Check sheet for the modelled part. Datum: model origin and axes. Units: mm. Face numbers are marked on the shaded views. Coordinates: 2 decimals unless noted, no trailing zeros. Loops run counter-clockwise (first coordinate to the right, second up) from the corner with the lowest first, then second, coordinate; pieces in that order, holes last.
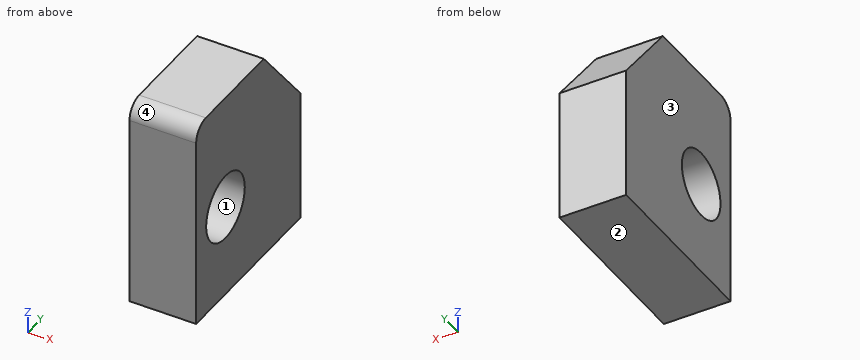
from build123d import *

# Parameters (mm, degrees)
F0_R     = 12.7
F1_DEPTH = 25.4


with BuildPart() as f1:
    # F0 (on Right) → F1 (new body)
    with BuildSketch(Plane.YZ):
        with BuildLine():
            Line((-8.451596, 44.603311), (-46.551596, 44.603311))
            ThreePointArc((-46.551596, 44.603311), (-51.041724, 42.743439), (-52.901596, 38.253311))
            Line((-52.901596, 38.253311), (-52.901596, -35.611195))
            Line((-52.901596, -35.611195), (15.764037, -35.611195))
            Line((15.764037, -35.611195), (15.764037, 15.188805))
            Line((15.764037, 15.188805), (-8.451596, 44.603311))
        make_face()
        with Locations((-33.608079, 0)):
            Circle(F0_R, mode=Mode.SUBTRACT)
    extrude(amount=F1_DEPTH)


solid = f1.part
(1) Gauge pin test, flat ends, axial feed: P1, Ø4, axis at y = 4.5, z = 21, coming from the -X side; P2, Ø20.5, axis at y = -33.61, z = 0, coming from the +X side. Record the tip position at first contact, or that the pin passes through.
(2) Section check D-D, the plane z = 35.5. Enter the section's corners in (x, y), plus the area to 3 significant figures.
(3) Section check B-B, the plane x = 1.75. Enter the section's corners in (y, z), plus the area to 3 significant figures.
(4) Section check A-A, the plane z = 0. Enter the section's corners in (x, y), plus the area to 3 significant figures.
(5) Section check C-C, the plane y = -35.5. Enter the section's corners in (x, z), plus the area to 3 significant figures.
(6) Draft check along Z on the marked faces 1, 2, 3 and 4. Enter one of: pulls with the +Z half, pulls with the -Z half, needs draft (parallel to the pull), parting line crosses it, or undercut.
(7) Scan lines: line 1 along Z through (x, y) = (18.25, -33); line 2 along Z through (x, y) = (12.25, -43); line 3 along Y through (x, z) = (12.5, -2). Record each from-to range of solid material in increasing order.
Determined:
1. P1: stops at x = 0
1. P2: passes through
2. outline: (0, -52.9) - (25.4, -52.9) - (25.4, -0.96) - (0, -0.96) - close
2. area: 1,320 mm2
3. outline: (-52.9, -35.61) - (15.76, -35.61) - (15.76, 15.19) - (-8.45, 44.6) - (-46.55, 44.6) arc R6.35 ccw to (-52.9, 38.25) - close; hole circle Ø25.4 at (-33.61, 0)
3. area: 4,640 mm2
4. outline: (0, -52.9) - (25.4, -52.9) - (25.4, -46.31) - (0, -46.31) - close; (0, -20.91) - (25.4, -20.91) - (25.4, 15.76) - (0, 15.76) - close
4. area: 1,100 mm2
5. outline: (0, -35.61) - (25.4, -35.61) - (25.4, -12.56) - (0, -12.56) - close; (0, 12.56) - (25.4, 12.56) - (25.4, 44.6) - (0, 44.6) - close
5. area: 1,400 mm2
6. face 1: undercut
6. face 2: pulls with the -Z half
6. face 3: needs draft
6. face 4: pulls with the +Z half
7. line 1: z = -35.61 to -12.69, 12.69 to 44.6
7. line 2: z = -35.61 to -8.55, 8.55 to 44.6
7. line 3: y = -52.9 to -46.15, -21.07 to 15.76
